The figure shows three views and two pictorial views of one solid part (mm, origin at its lowest corner). Answer the questions. Round coordinates to 2 decimals unless told otherwise and drop trailing zeros. Order: outer loops, then holes, each group sorted by start corner. A loop starts at its lowest first (then second) coordinate and runs counter-clockwise, first axis right, second up. Notation, with made-up numbers: M 52.5,86.25 L 111.5,86.25 A24 ccw 111.5,123.25 Z; hole C 55,42 d3. An arc over 180 degrees is marked long. Answer as CSV lines item,"result".
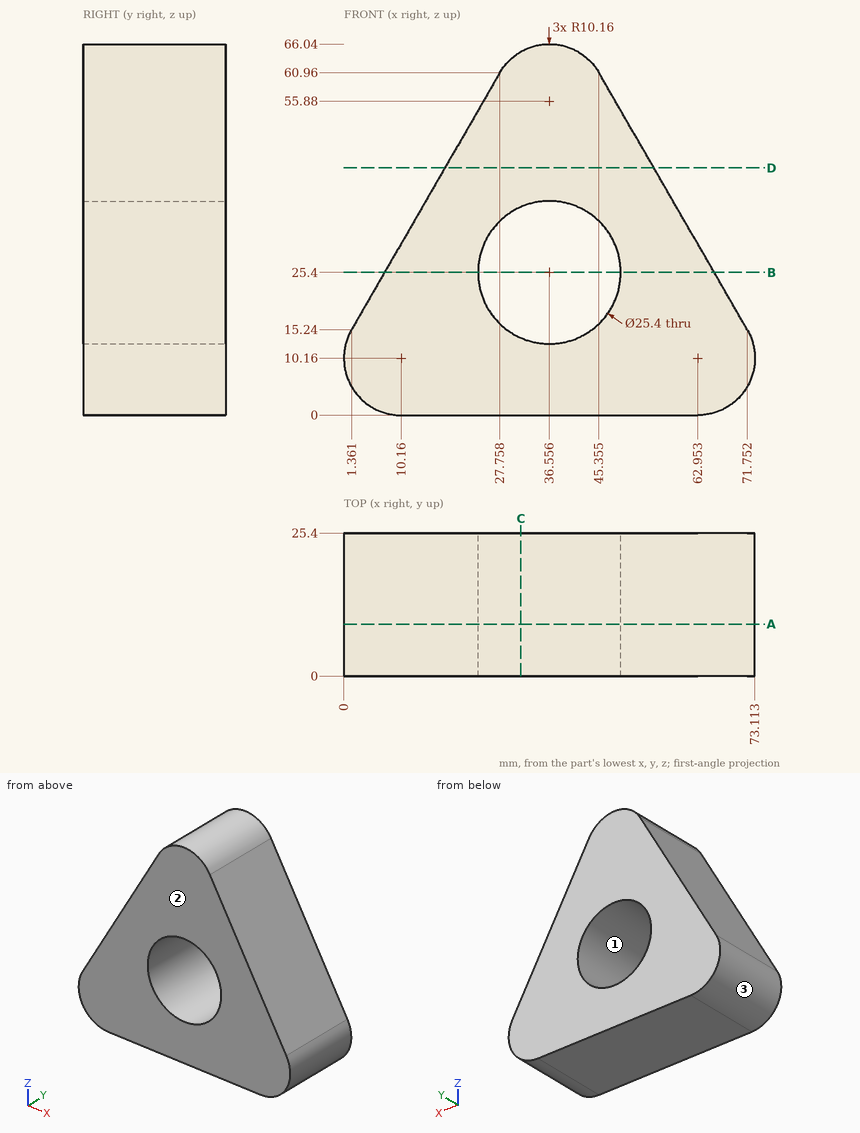
Item 1: A cutting plane is placed at A-A, the plane y = 9.25. Determine the outline of the cut face in (x, z) (1 decimal).
Ans:
outline,"M 1.4,15.2 A10.2 ccw 10.2,0 L 63,0 A10.2 ccw 71.8,15.2 L 45.4,61 A10.2 ccw 27.8,61 Z; hole C 36.6,25.4 d25.4"
Item 2: Flat-ended cylindrical pins translate along their axes: pin 1 (8 mm diameter, centred on y = 20, z = 18.5, fed in from +X); pin 2 (1 mm diameter, centred on y = 20.5, z = 15.5, fed in from +X) (1 decimal); pin 3 (6 mm diameter, centred on x = 59.5, y = 11, fed in from +Z) (1 decimal). Find the tip coordinate at first contact, or state that the pin passes through.
Ans:
pin 1,"x = 72.14"
pin 2,"x = 71.9"
pin 3,"z = 41.7"
Item 3: Find the intervals of material crossed by probe 1 along Z at (x, y) = (46, 21.5) (1 decimal); probe 2 along Z at (x, y) = (31, 13) (1 decimal); probe 3 along X at (y, z) = (6.5, 10), in increasing order. Write a range as [from, to].
Ans:
probe 1,"[0, 16.9], [33.9, 59.8]"
probe 2,"[0, 14], [36.8, 64.4]"
probe 3,"[0, 73.11]"
Item 4: A cutting plane is placed at B-B, the plane z = 25.4. Determine the outline of the cut face in (x, y) (1 decimal).
Ans:
outline,"M 7.2,0 L 23.9,0 L 23.9,25.4 L 7.2,25.4 Z; M 49.3,0 L 65.9,0 L 65.9,25.4 L 49.3,25.4 Z"
Item 5: Determine the mould class of the marked faces 1, 2 and 3 for opening direction Z: +Z half, -Z half, draft (parallel to the pull), parting line (faces both ways), or undercut.
Ans:
face 1,"undercut"
face 2,"draft"
face 3,"parting line"
Item 6: A cutting plane is placed at D-D, the plane z = 44. Determine the outline of the cut face in (x, y) (1 decimal).
Ans:
outline,"M 18,0 L 55.1,0 L 55.1,25.4 L 18,25.4 Z"
Item 7: A cutting plane is placed at C-C, the plane x = 31.5. Determine the outline of the cut face in (y, z), and give its area (3 significant figures).
Ans:
outline,"M 0,0 L 25.4,0 L 25.4,13.75 L 0,13.75 Z; M 0,37.05 L 25.4,37.05 L 25.4,64.69 L 0,64.69 Z"
area,"1,050 mm2"
